```python
from build123d import *

# Parameters (mm, degrees)
SKETCH_1_R      = 12.5
SKETCH_1_R_2    = 7.5
EXTRUDE_1_DEPTH = 10
EXTRUDE_3_DEPTH = 5
SKETCH_1_5_R    = 6
SKETCH_1_5_R_2  = 4
EXTRUDE_4_DEPTH = 4


with BuildPart() as part:
    # Sketch 1 → Extrude 1 (new body)
    with BuildSketch(Plane(origin=(0, 0, 0), x_dir=(1, 0, 0), z_dir=(0, 1, 0))):
        with Locations(Location((0, 0, 0), (0, 0, 270))):
            Circle(SKETCH_1_R)
        with Locations(Location((0, 0, 0), (0, 0, 270))):
            Circle(SKETCH_1_R_2, mode=Mode.SUBTRACT)
    extrude(amount=EXTRUDE_1_DEPTH)

    # Sketch 1_4 → Extrude 3 (add)
    with BuildSketch(Plane(origin=(0, 0, 0), x_dir=(1, 0, 0), z_dir=(0, 1, 0))):
        with BuildLine():
            ThreePointArc((0, -12.5), (-12.5, 0), (0, 12.5))
            Line((0, 12.5), (-30, 12.5))
            Line((-30, 12.5), (-30, 6.5))
            Line((-30, 6.5), (-17, 6.5))
            Line((-17, 6.5), (-17, -6.5))
            Line((-17, -6.5), (-30, -6.5))
            Line((-30, -6.5), (-30, -12.5))
            Line((-30, -12.5), (0, -12.5))
        make_face()
    extrude(amount=EXTRUDE_3_DEPTH)

    # Sketch 1_5 → Extrude 4 (add)
    # profile 1 of 2: a face of its own
    with BuildSketch(Plane(origin=(0, 0, 0), x_dir=(1, 0, 0), z_dir=(0, 1, 0))):
        with BuildLine():
            Line((20.301898362, 16.813158484), (8.321859729, 9.327199507))
            ThreePointArc((8.321859729, 9.327199507), (10.600601202, 6.623990803), (12.031294579, 3.390862834))
            Line((12.031294579, 3.390862834), (24.011333212, 10.876821811))
            ThreePointArc((24.011333212, 10.876821811), (21.201202404, 13.247981606), (20.301898362, 16.813158484))
        make_face()
    # profile 2 of 2: a face of its own
    with BuildSketch(Plane(origin=(0, 0, 0), x_dir=(1, 0, 0), z_dir=(0, 1, 0))):
        with Locations((26.289490981, 16.427497191)):
            Circle(SKETCH_1_5_R)
        with Locations(Location((26.289490981, 16.427497191, 0), (0, 0, 270))):
            Circle(SKETCH_1_5_R_2, mode=Mode.SUBTRACT)
    extrude(amount=EXTRUDE_4_DEPTH)


solid = part.part
```
The model under review builds one solid part; all positions refer to its coordinate system, in mm. A direction names the side the tool comes from. Round coordinates to 2 decimals unless told otherwise and drop trailing zeros. Loops run counter-clockwise (first coordinate to the right, second up) from the corner with the lowest first, then second, coordinate; pieces in that order, holes last. Notation, with made-up numbers: M 62.5,-9.5 L 74.5,-9.5 A31 cw 74.5,27.5 Z; hole C 15.25,89 d5. An arc over 180 degrees is marked long. Put each result on its own line as item: value.
Q1. Mouldability with a two-part tool opening along Z and no side actions: class faces 5 (the cylindrical face through (31.5, 2, -19.4)), 6 (the flat face through (-30, 2, 9)), 7 (the cylindrical face through (0.33, 4.93, -7.493)) as released by +Z, released by -Z, zero draft, split by the parting line, or undercut.
Result set:
face 5: split by the parting line
face 6: zero draft
face 7: undercut
Q2. Consider section D-D, the plane x = 21. Give the boundary of the cut face in (y, z).
Result set:
outline: M 0,-19.26 L 4,-19.26 L 4,-9 L 0,-9 Z
Q3. To check wall thickness, follow L1, parallel to Z at x = -18, y = 0.5; L2, parallel to X at y = 4.5, z = 0; L3, parallel to X at y = 6.75, z = 0. State the ranges of each line that lie inside material, in increasing order.
Result set:
L1: z = -12.5 to -6.5, 6.5 to 12.5
L2: x = -17 to -7.5, 7.5 to 12.5
L3: x = -12.5 to -7.5, 7.5 to 12.5
Q4. Consider section C-C, the plane y = 6. Give the boundary of the cut face in (x, z).
Result set:
outline: C 0,0 d25; hole C 0,0 d15
Q5. Consider section A-A, the plane z = 0. Give the boundary of the cut face in (x, y), then the cut area to 4 significant figures.
Result set:
outline: M -17,0 L -7.5,0 L -7.5,10 L -12.5,10 L -12.5,5 L -17,5 Z; M 7.5,0 L 12.5,0 L 12.5,10 L 7.5,10 Z
area: 122.5 mm²
Q6. Consider section B-B, the plane y = 1. Give the boundary of the cut face in (x, z), then the cut area to 3 significant figures.
Result set:
outline: M -30,-12.5 L 0,-12.5 A12.5 ccw 8.32,-9.33 L 20.3,-16.81 A6 ccw long 24.01,-10.88 L 12.03,-3.39 A12.5 ccw 0,12.5 L -30,12.5 L -30,6.5 L -17,6.5 L -17,-6.5 L -30,-6.5 Z; hole C 0,0 d15; hole C 26.29,-16.43 d8
area: 804 mm²
Q7. For pin 1 (5 mm diameter, centred on x = -5.5, y = 5, fed in from -Z); pin 2 (1.5 mm diameter, centred on y = 3, z = 1.5, fed in from -X); pin 3 (4 mm diameter, centred on x = 15.5, y = 5.5, fed in from -Z), all flat-tipped, find the tip position at first contact; note any pin that passes through.
Result set:
pin 1: stops at z = -12.5
pin 2: stops at x = -17
pin 3: stops at z = -14.64
Q8. Machinability: for faces 1 (the flat face through (-15, 2, -12.5)), 2 (the flat face through (20, 4, -12)), 3 (the cylindrical face through (12.394, 6.041, -1.627)), 4 (the flat face through (-17, 2, 0)), which of the approach directions +Z, -Z, +X, -X, +Y, -Y give a long, thin tool a straight path to every point of the face, cutting with its end or side? Answer none if there is none.
Result set:
face 1: -Z, -X, +Y, -Y
face 2: -Z, +X, +Y
face 3: +Y
face 4: -X, +Y, -Y
